```python
from build123d import *

# Parameters (mm, degrees)
SKETCH_1_R      = 5
EXTRUDE_1_DEPTH = 5
SKETCH_1_6_W    = 10
SKETCH_1_6_H    = 5
EXTRUDE_3_DEPTH = 20
EXTRUDE_START   = 15
SKETCH_1_7_W    = 10
SKETCH_1_7_H    = 5
EXTRUDE_4_DEPTH = 5


with BuildPart() as part:
    # Sketch 1 → Extrude 1 (new body)
    with BuildSketch(Plane.XY):
        with BuildLine():
            ThreePointArc((10, 10), (0, 20), (-10, 10))
            Line((-10, 10), (-20, 10))
            Line((-20, 10), (-20, 0))
            Line((-20, 0), (10, 0))
            Line((10, 0), (10, 10))
        make_face()
        with Locations((0, 10)):
            Circle(SKETCH_1_R, mode=Mode.SUBTRACT)
    extrude(amount=EXTRUDE_1_DEPTH)

    # Sketch 1_6 → Extrude 3 (add)
    with BuildSketch(Plane.XY):
        Polygon((10, 0), (10, 5), (0, 5), (-10, 5), (-10, 0), align=None)
        with Locations((-15, 2.5)):
            Rectangle(SKETCH_1_6_W, SKETCH_1_6_H)
    extrude(amount=EXTRUDE_3_DEPTH)

    # Sketch 1_7 → Extrude 4 (add)
    with BuildSketch(Plane.XY.offset(EXTRUDE_START)):
        with BuildLine():
            Line((-20, 10), (-10, 10))
            ThreePointArc((-10, 10), (-13.535533906, 11.464466094), (-15, 15))
            Line((-15, 15), (-20, 15))
            Line((-20, 15), (-20, 10))
        make_face()
        with Locations((-15, 7.5)):
            Rectangle(SKETCH_1_7_W, SKETCH_1_7_H)
    extrude(amount=EXTRUDE_4_DEPTH)


solid = part.part
```
Could you check a few things on this model? Use its own coordinates, in mm. A direction names the side the tool comes from. Coordinates: 2 decimals unless noted, no trailing zeros. Order: outer loops, then holes, each group sorted by start corner. A loop starts at its lowest first (then second) coordinate and runs counter-clockwise, first axis right, second up. Notation, with made-up numbers: M 26.5,47 L 83.5,47 A28 cw 83.5,73 Z; hole C 8.5,22.25 d4. An arc over 180 degrees is marked long. Use a Markdown table: item, result. Add a question column.
Q1. We'd pull the mould along Y, two halves only. Please class faces 1 (the cylindrical face through (-0.651, 14.957, 2.465)), 2 (the flat face through (-9, 4, 20)), 3 (the cylindrical face through (0, 20, 2)): pulls with the +Y half, pulls with the -Y half, needs draft (parallel to the pull), parting line crosses it, or undercut.
Q2. I want a section at A-A on y = 12.5. List the corners of the cut face in (x, z) for me.
Q3. Which directions (+Z, -Z, +X, -X, +Y, -Y) give clear straight access to the entire face, cutting with the end or side of a thin tool? Please do faces 4 (the flat face through (-5.2, 10.9, 5)), 5 (the flat face through (-15, 10, 2)), 6 (the flat face through (-10, 7, 17)).
Q4. I'm going to push flat-ended pins straight in: pin 1 (4 mm diameter, centred on x = -5, y = 8, fed in from +Z); pin 2 (4.5 mm diameter, centred on x = 2, z = 10, fed in from +Y); pin 3 (2.5 mm diameter, centred on x = -17.5, z = 17, fed in from +Y). Where does each tip first touch, or does it pass through?
Q5. I want a section at C-C on x = -3.5. List the corners of the cut face in (y, z) for me, then the cut area to 3 significant figures.
Q6. I want a section at B-B on z = 2.75. List the corners of the cut face in (x, y) for me.
Q7. I want a section at D-D on z = 15.75. List the corners of the cut face in (x, y) for me, then the cut area to 3 significant figures.
Q8. If I drill on L1, parallel to Y at x = 0, z = 3.35; L2, parallel to Y at x = -1, z = 18.75, over which ranges is the centre line in solid material (lowest first)?
Checked values:
| question | item | result |
|---|---|---|
| 1 | face 1 | undercut |
| 1 | face 2 | needs draft |
| 1 | face 3 | pulls with the +Y half |
| 2 | outline | M -20,15 L -14.33,15 L -14.33,20 L -20,20 Z; M -9.68,0 L -4.33,0 L -4.33,5 L -9.68,5 Z; M 4.33,0 L 9.68,0 L 9.68,5 L 4.33,5 Z |
| 3 | face 4 | +X, -X, +Y |
| 3 | face 5 | -Z, -X, +Y |
| 3 | face 6 | +Z, +X, +Y |
| 4 | pin 1 | z = 5 |
| 4 | pin 2 | y = 5 |
| 4 | pin 3 | y = 15 |
| 5 | outline | M 0,0 L 6.43,0 L 6.43,5 L 5,5 L 5,20 L 0,20 Z; M 13.57,0 L 19.37,0 L 19.37,5 L 13.57,5 Z |
| 5 | area | 136 mm² |
| 6 | outline | M -20,0 L 10,0 L 10,10 A10 ccw -10,10 L -20,10 Z; hole C 0,10 d10 |
| 7 | outline | M -20,0 L 10,0 L 10,5 L -10,5 L -10,10 A5 cw -15,15 L -20,15 Z |
| 7 | area | 230 mm² |
| 8 | L1 | 0 to 5, 15 to 20 |
| 8 | L2 | 0 to 5 |
